```python
from build123d import *

# Parameters (mm, degrees)
SKETCH1_R             = 6.35
SKETCH1_R_2           = 3.175
BOSS_EXTRUDE1_DEPTH   = 1.5875
F_4_CLEARANCE_HOLE1_D = 3.2639


with BuildPart() as part:
    # Sketch1 → Boss-Extrude1 (new body, symmetric)
    with BuildSketch(Plane.XY):
        with BuildLine():
            Line((49.048701781, -45.301306076), (49.048701781, 17.681627212))
            Line((49.048701781, 17.681627212), (6.35250271, 34.342413053))
            ThreePointArc((6.35250271, 34.342413053), (-21.3593907, 27.632083778), (-34.835067544, 2.504734358))
            ThreePointArc((-34.835067544, 2.504734358), (-30.426385746, -2.587056811), (-25.334594577, 1.821624988))
            ThreePointArc((-25.334594577, 1.821624988), (1.502184662, 25.355540642), (25.372459089, -1.182505722))
            ThreePointArc((25.372459089, -1.182505722), (18.055035291, -29.123378386), (0, -51.667840164))
            Line((0, -51.667840164), (0, -92.444233417))
            ThreePointArc((0, -92.444233417), (6.35, -86.094233417), (12.7, -92.444233417))
            ThreePointArc((12.7, -92.444233417), (10.290303985, -97.423842288), (4.89007732, -98.624130323))
            ThreePointArc((4.89007732, -98.624130323), (8.832322877, -101.466501446), (9.610051547, -106.263949908))
            ThreePointArc((9.610051547, -106.263949908), (13.067449766, -103.840245814), (15.875, -106.993911248))
            ThreePointArc((15.875, -106.993911248), (15.780924606, -107.761067405), (15.504273342, -108.482761819))
            Line((15.504273342, -108.482761819), (49.048701781, -45.301306076))
        make_face()
        with Locations((6.35, -92.444233417)):
            Circle(SKETCH1_R)
        with Locations((12.7, -106.993911248)):
            Circle(SKETCH1_R_2)
    extrude(amount=BOSS_EXTRUDE1_DEPTH, both=True)

    # #4 Clearance Hole1 (through all)
    with Locations(Plane.XY.offset(1.5875)):
        with Locations((12.7, -106.993911248)):
            Hole(F_4_CLEARANCE_HOLE1_D / 2)


solid = part.part
```
The listing builds one solid part. Answer for the finished solid, in the listing's coordinates (mm). A direction names the side the tool comes from. Give positions to 0.01 mm unless a question says otherwise; leave off trailing zeros. Order: outer loops, then holes, each group sorted by start corner. A loop starts at its lowest first (then second) coordinate and runs counter-clockwise, first axis right, second up. Notation, with made-up numbers: (45.25, 75) -> (94.25, 75) arc R17 cw to (94.25, 93) -> close; hole circle Ø1 at (76.25, 6). An arc over 180 degrees is marked (long way). Answer as a JSON object with one key per item and string values. Group by question number.
Item 1: The part is cut by section C-C on y = -82. Write down the section's boundary in (x, z).
Item 2: Consider L1, parallel to Y at x = 12.7, z = 0.15; L2, parallel to X at y = 0.5, z = 0.45; L3, parallel to Y at x = 2.5, z = -0.2. Determine where each line is inside the solid, lowest interval first. Write a range as from..to.
Item 3: The part is cut by section A-A on x = 19.5. Write down the section's boundary in (y, z).
Item 4: A flat-ended cylindrical pin translates along its axis: pin 1 (8 mm diameter, centred on x = 7.5, y = 19, fed in from +Z). Find the tip coordinate at first contact, or state that the pin passes through.
Item 5: Determine the mould class of faces 1 (the flat face through (27.999, 25.895, 0.022)), 2 (the flat face through (0, -72, 0)), 3 (the flat face through (25, -37, -1.588)), 4 (the cylindrical face through (12.912, -105.376, -0.022)) for opening direction X: pulls with the +X half, pulls with the -X half, needs draft (parallel to the pull), parting line crosses it, or undercut.
Item 6: A tool of negligible diameter and unlimited length cuts with its end or side. For faces 5 (the cylindrical face through (0.949, 25.382, 0.022)), 6 (the flat face through (49.049, -14, 0)), from which of +Z, -Z, +X, -X, +Y, -Y can it reach the whole face along a straight path? Write none if from no direction.
Result set:
{
 "1": {"outline": "(0, -1.59) -> (29.56, -1.59) -> (29.56, 1.59) -> (0, 1.59) -> close"},
 "2": {"L1": "-110.17..-108.63, -105.36..-38.04, 22..31.87", "L2": "-34.55..-25.62, 25.4..49.05", "L3": "-97.49..-49.52, 25.28..34.84"},
 "3": {"outline": "(-100.96, -1.59) -> (-26.06, -1.59) -> (-26.06, 1.59) -> (-100.96, 1.59) -> close; (16.28, -1.59) -> (29.21, -1.59) -> (29.21, 1.59) -> (16.28, 1.59) -> close"},
 "4": {"pin 1": "through"},
 "5": {"face 1": "pulls with the +X half", "face 2": "pulls with the -X half", "face 3": "needs draft", "face 4": "undercut"},
 "6": {"face 5": "+Z, -Z", "face 6": "+Z, -Z, +X, +Y, -Y"}
}
